Read the model definition and answer for the solid it produces. Units are mm, in the model's axes. A direction names the side the tool comes from. Round coordinates to 2 decimals unless told otherwise and drop trailing zeros. Order: outer loops, then holes, each group sorted by start corner. A loop starts at its lowest first (then second) coordinate and runs counter-clockwise, first axis right, second up. Notation, with made-up numbers: (14.5, 54) - (56.5, 54) arc R27 ccw to (56.5, 89) - close; hole circle Ø6 at (88, 60.5). An arc over 180 degrees is marked (long way). One line per question, with ' | ' between items. Start each with the question number.
1) The part is cut by section B-B, the plane x = 75. Give the vertices of the cut face in (y, z) (3 decimals).
2) The part is cut by section A-A, the plane y = 21.25. Give the vertices of the cut face in (x, z), plus the area to 3 significant figures.
3) The part is cut by section D-D, the plane x = 43.81. Give the vertices of the cut face in (y, z).
4) For faces 5 (the cylindrical face through (107.465, 5.903, -34.169)), 6 (the flat face through (85, 7, -6.825)), 7 (the flat face through (85, 13.285, -7)), 8 (the flat face through (30, 17.1, -5)), 9 (the flat face through (108, 25, -19)), determine the directions among +Z, -Z, +X, -X, +Y, -Y from which every point of the face is accessible in a straight line to the end or side of a thin tool.
5) The part is cut by section C-C, the plane z = -5. Count the separate pieces of the cut face and the enclosed holes in it, plus the area to 3 significant figures.
6) Straight lines are drawn through the part: line 1 (X direction, y = 19.5, z = -5); line 2 (X direction, y = 2.5, z = -5) (3 decimals); line 3 (Y direction, x = 37, z = -8.5). For each, find the intervals that lie inside material, in ascending order. Write a range as from..to.
7) The mould has two halves that part along X. Classify faces 1 (the flat face through (60, 13, -5)), 2 (the cylindrical face through (3.403, 3.895, -4.169)), 3 (the cylindrical face through (42.053, 3.895, -5.39)), 4 (the cylindrical face through (107.465, 5.903, -24.169)): pulls with the +X half, pulls with the -X half, needs draft (parallel to the pull), parting line crosses it, or undercut.
8) Flat-ended cylindrical pins translate along their axes: pin 1 (5 mm diameter, centred on x = 18.5, z = -6, fed in from -Y); pin 2 (3 mm diameter, centred on y = 17.5, z = -25, fed in from +X); pin 3 (7.5 mm diameter, centred on x = 41, y = 8.5, fed in from -Z); pin 4 (5 mm diameter, centred on y = 7.5, z = -29.5, fed in from -X). Find the tip coordinate at first contact, or state that the pin passes through.
from build123d import *

# Parameters (mm, degrees)
SKETCH1_W           = 110
SKETCH1_H           = 10
SKETCH1_R           = 1.8
BOSS_EXTRUDE1_DEPTH = 25
SKETCH2_W           = 10
SKETCH2_H           = 9.2
CUT_EXTRUDE1_DEPTH  = 60
SKETCH16_W          = 5
SKETCH16_H          = 25
BOSS_EXTRUDE2_DEPTH = 10
SKETCH17_R          = 1.8
CUT_EXTRUDE6_DEPTH  = 10
SKETCH18_W          = 5
SKETCH18_H          = 25
BOSS_EXTRUDE3_DEPTH = 20
SKETCH19_R          = 1.8
CUT_EXTRUDE7_DEPTH  = 12
SKETCH20_W          = 5
SKETCH20_H          = 2.078520269
CUT_EXTRUDE8_DEPTH  = 46
SKETCH21_W          = 40
SKETCH21_H          = 10
CUT_EXTRUDE9_DEPTH  = 11.715
CUT_EXTRUDE10_DEPTH = 13.285


with BuildPart() as part:
    # Sketch1 → Boss-Extrude1 (new body)
    with BuildSketch(Plane(origin=(0, 0, 0), x_dir=(1, 0, 0), z_dir=(0, 1, 0))):
        with Locations((55, 5)):
            Rectangle(SKETCH1_W, SKETCH1_H)
        with Locations(Location((5, 5, 0), (0, 0, 270))):
            Circle(SKETCH1_R, mode=Mode.SUBTRACT)
        with Locations(Location((43.81, 5, 0), (0, 0, 270))):
            Circle(SKETCH1_R, mode=Mode.SUBTRACT)
    extrude(amount=BOSS_EXTRUDE1_DEPTH)

    # Sketch2 → Cut-Extrude1 (cut)
    with BuildSketch(Plane.ZY):
        with Locations((-5, 12.5)):
            Rectangle(SKETCH2_W, SKETCH2_H)
    extrude(amount=-CUT_EXTRUDE1_DEPTH, mode=Mode.SUBTRACT)

    # Sketch16 → Boss-Extrude2 (add)
    with BuildSketch(Plane(origin=(0, 0, -10), x_dir=(-1, 0, 0), z_dir=(0, 0, -1))):
        with Locations((-107.5, 12.5)):
            Rectangle(SKETCH16_W, SKETCH16_H)
    extrude(amount=BOSS_EXTRUDE2_DEPTH)

    # Sketch17 → Cut-Extrude6 (cut)
    with BuildSketch(Plane(origin=(110, 0, 0), x_dir=(0, 0, -1), z_dir=(1, 0, 0))):
        with Locations((15, 7.5)):
            Circle(SKETCH17_R)
        with Locations((15, 17.5)):
            Circle(SKETCH17_R)
    extrude(amount=-CUT_EXTRUDE6_DEPTH, mode=Mode.SUBTRACT)

    # Sketch18 → Boss-Extrude3 (add)
    with BuildSketch(Plane(origin=(0, 0, -20), x_dir=(-1, 0, 0), z_dir=(0, 0, -1))):
        with Locations((-107.5, 12.5)):
            Rectangle(SKETCH18_W, SKETCH18_H)
    extrude(amount=BOSS_EXTRUDE3_DEPTH)

    # Sketch19 → Cut-Extrude7 (cut)
    with BuildSketch(Plane.ZY.offset(-105)):
        with Locations((-25, 17.5)):
            Circle(SKETCH19_R)
        with Locations((-25, 7.5)):
            Circle(SKETCH19_R)
        with Locations((-35, 17.5)):
            Circle(SKETCH19_R)
        with Locations((-35, 7.5)):
            Circle(SKETCH19_R)
    extrude(amount=-CUT_EXTRUDE7_DEPTH, mode=Mode.SUBTRACT)

    # Sketch20 → Cut-Extrude8 (cut)
    with BuildSketch(Plane.XZ):
        with Locations((107.5, -38.960739866)):
            Rectangle(SKETCH20_W, SKETCH20_H)
    extrude(amount=-CUT_EXTRUDE8_DEPTH, mode=Mode.SUBTRACT)

    # Sketch21 → Cut-Extrude9 (cut)
    with BuildSketch(Plane(origin=(0, 25, 0), x_dir=(1, 0, 0), z_dir=(0, 1, 0))):
        with Locations((85, 5)):
            Rectangle(SKETCH21_W, SKETCH21_H)
    extrude(amount=-CUT_EXTRUDE9_DEPTH, mode=Mode.SUBTRACT)

    # Sketch23 → Cut-Extrude10 (cut)
    with BuildSketch(Plane(origin=(0, 13.285, 0), x_dir=(1, 0, 0), z_dir=(0, 1, 0))):
        with BuildLine():
            Line((67.5, 6.825), (102.5, 6.825))
            ThreePointArc((102.5, 6.825), (104.325, 5), (102.5, 3.175))
            Line((102.5, 3.175), (67.5, 3.175))
            ThreePointArc((67.5, 3.175), (65.675, 5), (67.5, 6.825))
        make_face()
    extrude(amount=-CUT_EXTRUDE10_DEPTH, mode=Mode.SUBTRACT)


solid = part.part
Values:
1) outline: (0, -10) - (13.285, -10) - (13.285, -6.825) - (0, -6.825) - close; (0, -3.175) - (13.285, -3.175) - (13.285, 0) - (0, 0) - close
2) outline: (0, -10) - (65, -10) - (65, 0) - (0, 0) - close; (105, -37.92) - (110, -37.92) - (110, 0) - (105, 0) - close; hole circle Ø3.6 at (5, -5); hole circle Ø3.6 at (43.81, -5) | area: 819 mm^2
3) outline: (0, -10) - (7.9, -10) - (7.9, -6.8) - (0, -6.8) - close; (0, -3.2) - (7.9, -3.2) - (7.9, 0) - (0, 0) - close; (17.1, -10) - (25, -10) - (25, -6.8) - (17.1, -6.8) - close; (17.1, -3.2) - (25, -3.2) - (25, 0) - (17.1, 0) - close
4) face 5: +X, -X | face 6: +Y, -Y | face 7: +Z, -Z, +Y | face 8: +Z, -Z, -X | face 9: +Z, -Z, +X, -X, +Y
5) separate pieces: 6 | enclosed holes: 0 | area: 1,100 mm^2
6) line 1: x = 0..3.2, 6.8..42.01, 45.61..65, 105..110 | line 2: x = 0..3.2, 6.8..42.01, 45.61..65.675, 104.325..110 | line 3: y = 0..7.9, 17.1..25
7) face 1: pulls with the -X half | face 2: undercut | face 3: undercut | face 4: needs draft
8) pin 1: stops at y = 0 | pin 2: passes through | pin 3: stops at z = -10 | pin 4: stops at x = 105
